The model under review builds one solid part; all positions refer to its coordinate system, in mm. Face numbers are marked on the shaded views. A direction names the side the tool comes from. Round coordinates to 2 decimals unless told otherwise and drop trailing zeros. Order: outer loops, then holes, each group sorted by start corner. A loop starts at its lowest first (then second) coordinate and runs counter-clockwise, first axis right, second up. Notation, with made-up numbers: M 58.5,23 L 94.5,23 A11 cw 94.5,28 Z; hole C 56,40.25 d11. An arc over 180 degrees is marked long. Answer as a JSON object with one key per item and string values. Group by question number.
1. Clearance check with flat-ended pins moving along their axes: P1, Ø6, axis at x = 31.76, y = -14.06, coming from the +Z side (3 decimals); P2, Ø8, axis at x = 18.55, y = -1.36, coming from the -Z side; P3, Ø8, axis at x = 15.172, z = 25.4, coming from the -Y side; P4, Ø10, axis at y = -1.5, z = 53, coming from the +X side. State where each tip first meets the part, or that it passes through.
2. Add section D-D on z = 25.4. State the section outline as (x, y) points (3 decimals).
3. Add section A-A on x = 7. Give the number of separate pieces and of enclosed holes in the cut face, and give its area (3 significant figures).
4. To check wall thickness, follow probe 1 along X at (y, z) = (10, 12); probe 2 along Z at (x, y) = (13, -19) (3 decimals); probe 3 along X at (y, z) = (-11.5, 65.5). State the ranges of each line that lie inside material, in increasing order. Write a range as [from, to].
5. Add section B-B on y = 4.5. State the section outline as (x, z) points (3 decimals), and give its area (3 significant figures).
6. Machinability: for the marked faces 1, 2 and 3, which of the approach directions +Z, -Z, +X, -X, +Y, -Y give a long, thin tool a straight path to every point of the face, cutting with its end or side? Answer none if there is none.
7. Add section C-C on z = 37. State the section outline as (x, y) points (3 decimals).
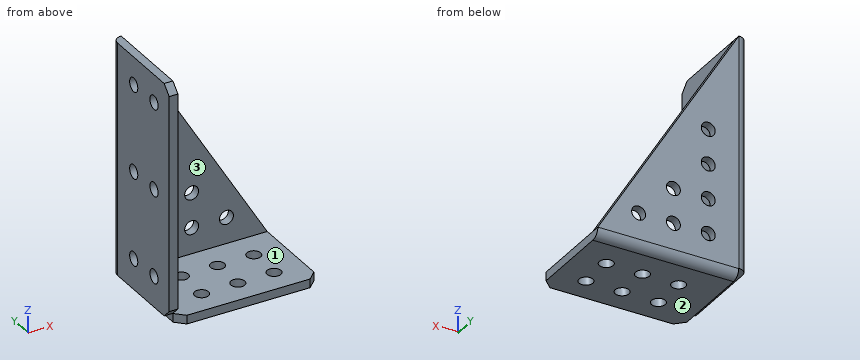
Autodesk Inventor part; units mm, degrees
ref_plane "YZ Plane" through (0, 0, 0) normal (1, 0, 0) x (0, 1, 0)
ref_plane "XZ Plane" through (0, 0, 0) normal (0, 1, 0) x (-1, 0, 0)
ref_plane "XY Plane" through (0, 0, 0) normal (0, 0, 1) x (1, 0, 0)
sketch "Sketch1" plane through (0, 0, 0) normal (0, 0, 1) x (1, 0, 0)
  line L0 (-11.879, 12.2271) -> (42.731, 12.2271)
  line L1 (42.731, 12.2271) -> (42.731, -23.3329)
  line L2 (42.731, -23.3329) -> (-11.879, -23.3329)
  line L3 (-11.879, -23.3329) -> (-11.879, 12.2271)
  point P0 (0, 0)
  dimension "d0" = 54.61
  dimension "d1" = 35.56
extrude "Extrusion1" add sketch "Sketch1" along normal blind 88.1634
sketch "Sketch5" plane through (42.731, -23.3329, 0) normal (1, 0, 0) x (0, 0, -1)
  line L0 (0, 35.56) -> (0, 0)
  line L1 (0, 35.56) -> (-88.1634, 35.56)
  line L2 (-88.1634, 0) -> (-88.1634, 35.56)
  line L3 (0, 0) -> (-88.1634, 0)
  line L4 (-3.175, 32.385) -> (-88.1634, 32.385)
  line L5 (-3.175, 32.385) -> (-3.175, 0)
  point P0 (0, 23.3329)
  dimension "d7" = 3.175
  dimension "d8" = 3.175
extrude "Extrusion2" cut sketch "Sketch5" against normal blind 51.435 contours L3 L2 L4 L5
sketch "Sketch6" plane through (42.731, 9.0521, 3.175) normal (0, -1, 0) x (1, 0, 0)
  line L0 (0, 84.9884) -> (0, 0)
  line L1 (-51.435, 84.9884) -> (0, 84.9884)
  line L2 (-51.435, 84.9884) -> (0, 0)
  point P0 (-42.731, -3.175)
extrude "Extrusion3" cut sketch "Sketch6" against normal blind 51.435
sketch "Sketch7" plane through (-11.879, -23.3329, 0) normal (-1, 0, 0) x (0, 0, 1)
  line L0 (0, 0) -> (0, 35.56)
  line L1 (0, 0) -> (88.1634, 0)
  line L2 (0, 35.56) -> (88.1634, 35.56)
  line L3 (3.2512, 35.56) -> (3.2512, 0)
  point P0 (0, 23.3329)
  dimension "d13" = 3.2512
extrude "Extrusion4" cut sketch "Sketch7" against normal blind 3.2512
chamfer "Chamfer1" distance 3.175 angle 45 4 edges at (-10.2915, -23.3329, 88.1634) (-8.6278, -23.3329, 1.5875) (-10.2915, -23.3329, 3.2512) (42.731, -23.3329, 1.5875)
fillet "Fillet1" radius 3.175 2 edges at (-11.879, 12.2271, 45.7073) (17.0516, 12.2271, 0)
sketch "Sketch10" plane through (-8.6278, 9.0521, 3.175) normal (0, 0, 1) x (1, 0, 0)
  line L0 (51.3588, 0) -> (51.3588, -29.21)
  line L1 (51.3588, 0) -> (0, 0)
  line L2 (0, 0) -> (0, -29.21)
  line L3 (48.1838, -32.385) -> (3.175, -32.385)
  circle A0 centre (13.97, -10.414) radius 2.54
  circle A1 centre (13.97, -23.114) radius 2.54
  circle A2 centre (27.178, -10.414) radius 2.54
  circle A3 centre (27.178, -23.114) radius 2.54
  circle A4 centre (40.386, -10.414) radius 2.54
  circle A5 centre (40.386, -23.114) radius 2.54
  dimension "d46" = 5.08
  dimension "d47" = 10.414
  dimension "d50" = 12.7
  dimension "d53" = 13.208
  dimension "d56" = 13.97
sketch "Sketch8" plane through (-8.704, -23.3329, 0) normal (1, 0, 0) x (0, 0, -1)
  line L0 (-88.1634, 3.175) -> (-88.1634, 32.385)
  line L1 (-6.4262, 0) -> (-84.9884, 0)
  circle A0 centre (-78.0034, 9.525) radius 2.54
  circle A1 centre (-46.2534, 9.525) radius 2.54
  circle A2 centre (-14.5034, 9.525) radius 2.54
  circle A3 centre (-78.0034, 22.225) radius 2.54
  circle A4 centre (-46.2534, 22.225) radius 2.54
  circle A5 centre (-14.5034, 22.225) radius 2.54
  point P0 (0, 23.3329)
  dimension "d20" = 5.08
  dimension "d22" = 10.16
  dimension "d24" = 9.525
  dimension "d27" = 31.75
  dimension "d30" = 12.7
extrude "Extrusion5" cut sketch "Sketch8" against normal blind 3.2512
extrude "Extrusion6" cut sketch "Sketch10" against normal blind 25.4
sketch "Sketch12" plane through (-8.6278, 9.0521, 3.175) normal (0, -1, 0) x (1, 0, 0)
  line L0 (51.3588, 0) -> (0, 0)
  line L1 (-0.0762, 84.9884) -> (-0.0762, 0.0762)
  circle A0 centre (11.0998, 47.625) radius 2.54
  circle A1 centre (11.0998, 34.925) radius 2.54
  circle A2 centre (11.0998, 22.225) radius 2.54
  circle A3 centre (11.0998, 9.525) radius 2.54
  circle A4 centre (23.7998, 47.625) radius 2.54
  circle A5 centre (23.7998, 34.925) radius 2.54
  circle A6 centre (23.7998, 22.225) radius 2.54
  circle A7 centre (23.7998, 9.525) radius 2.54
  circle A8 centre (36.4998, 47.625) radius 2.54
  circle A9 centre (36.4998, 34.925) radius 2.54
  circle A10 centre (36.4998, 22.225) radius 2.54
  circle A11 centre (36.4998, 9.525) radius 2.54
  point P0 (8.6278, -3.175)
  dimension "d59" = 5.08
  dimension "d60" = 11.176
  dimension "d63" = 12.7
  dimension "d66" = 12.7
  dimension "d69" = 9.525
extrude "Extrusion7" cut sketch "Sketch12" against normal blind 25.4 contours A0 | A1 | A2 | A3 | A6 | A7 | A11
properties part number "Chassis_BumperAttachmentRight"
Recorded:
{
 "1": {"P1": "stops at z = 3.175", "P2": "stops at z = 0", "P3": "stops at y = 9.05", "P4": "stops at x = -8.7"},
 "2": {"outline": "M -11.879,-23.333 L -8.704,-23.333 L -8.704,9.052 L -0.068,9.052 L -0.068,12.227 L -8.704,12.227 A3.175 ccw -11.879,9.052 Z; M 5.012,9.052 L 12.632,9.052 L 12.632,12.227 L 5.012,12.227 Z; M 17.712,9.052 L 29.28,9.052 L 29.28,12.227 L 17.712,12.227 Z"},
 "3": {"separate pieces": "3", "enclosed holes": "0", "area": "274 mm²"},
 "4": {"probe 1": "x = [-11.73, 0.03], [4.91, 12.73], [17.61, 25.43], [30.31, 37.39]", "probe 2": "z = [0, 3.175]", "probe 3": "x = [-11.88, -8.7]"},
 "5": {"outline": "M -11.879,3.251 L -8.704,3.251 L -8.704,88.163 L -11.879,88.163 Z; M -8.628,0 L 42.731,0 L 42.731,3.175 L -8.628,3.175 Z", "area": "433 mm²"},
 "6": {"face 1": "+Z, +X, -X, -Y", "face 2": "-Z, +X, -X, +Y, -Y", "face 3": "+Z, +X, -Y"},
 "7": {"outline": "M -11.879,-23.333 L -8.704,-23.333 L -8.704,9.052 L 0.183,9.052 L 0.183,12.227 L -8.704,12.227 A3.175 ccw -11.879,9.052 Z; M 4.761,9.052 L 22.26,9.052 L 22.26,12.227 L 4.761,12.227 Z"}
}
